from build123d import *

# Parameters (mm, degrees)
SKETCH1_W                   = 304.8
SKETCH1_H                   = 63.5
BOSS_EXTRUDE1_DEPTH         = 9.525
F_1_4_20_TAPPED_HOLE1_D     = 5.1054
F_1_4_0_25_DIAMETER_HOLE1_D = 6.35
F_8_32_TAPPED_HOLE1_D       = 3.4544
F_8_32_TAPPED_HOLE1_DEPTH   = 14.986
F_8_32_TAPPED_HOLE1_TIP     = 1.037806461


with BuildPart() as part:
    # Sketch1 → Boss-Extrude1 (new body)
    with BuildSketch(Plane.XY):
        Rectangle(SKETCH1_W, SKETCH1_H)
    extrude(amount=BOSS_EXTRUDE1_DEPTH)

    # 1/4-20 Tapped Hole1 (through all)
    with Locations(Plane(origin=(-41.275, 23.114, 9.525), x_dir=(1, 0, 0), z_dir=(0, 0, 1))):
        with Locations((0, 0), (82.55, 0), (82.55, -38.1), (0, -38.1)):
            Hole(F_1_4_20_TAPPED_HOLE1_D / 2)

    # 1/4 (0.25) Diameter Hole1 (through all)
    with Locations(Plane(origin=(-117.475, 22.225, 9.525), x_dir=(1, 0, 0), z_dir=(0, 0, 1))):
        with Locations((0, 0), (0, -44.323), (234.823, -44.323), (234.823, 0)):
            Hole(F_1_4_0_25_DIAMETER_HOLE1_D / 2)

    # #8-32 Tapped Hole1
    with Locations(Plane(origin=(-139.7, 31.75, 4.445), x_dir=(0, 0, 1), z_dir=(0, 1, 0))):
        with Locations((0, 0), (0, 279.4)):
            Hole(F_8_32_TAPPED_HOLE1_D / 2, depth=F_8_32_TAPPED_HOLE1_DEPTH)
            with Locations((0, 0, -(F_8_32_TAPPED_HOLE1_DEPTH + F_8_32_TAPPED_HOLE1_TIP / 2))):  # 118° drill point
                Cone(0, F_8_32_TAPPED_HOLE1_D / 2, F_8_32_TAPPED_HOLE1_TIP, mode=Mode.SUBTRACT)


solid = part.part
Verification items for the finished model (mm, model axes). Round coordinates to 2 decimals unless told otherwise and drop trailing zeros. Order: outer loops, then holes, each group sorted by start corner. A loop starts at its lowest first (then second) coordinate and runs counter-clockwise, first axis right, second up. Notation, with made-up numbers: (-11.75, -4.5) -> (36.25, -4.5) arc R20 ccw to (36.25, 15.5) -> close; hole circle Ø3 at (36, 49.5). An arc over 180 degrees is marked (long way). Put each result on its own line as item: value.
1) Mould release check, pull along X, two halves, no side actions. Record for faces 1 (the flat face through (-2, -31.75, 5)), 2 (the flat face through (-152.4, 0, 5)), 3 (the cylindrical face through (38.84, -14.22, 4.7)): +X half, -X half, draft (parallel to the pull), parting line (faces both ways), or undercut.
Final values:
face 1: draft
face 2: -X half
face 3: undercut
2) Depth check by flat-ended pin: pin 1 (6 mm diameter, centred on x = 41.275, y = 23.114, fed in from +Z) (3 decimals); pin 2 (3 mm diameter, centred on x = -139.7, z = 4.445, fed in from +Y). Enter the tip coordinate at first touch or a pass-through.
Final values:
pin 1: stops at z = 9.525
pin 2: stops at y = 16.63
3) Section check A-A (x = 117.5). Record the cut outline in (y, z) (3 decimals).
Final values:
outline: (-31.75, 0) -> (-25.269, 0) -> (-25.269, 9.525) -> (-31.75, 9.525) -> close; (-18.927, 0) -> (19.054, 0) -> (19.054, 9.525) -> (-18.927, 9.525) -> close; (25.396, 0) -> (31.75, 0) -> (31.75, 9.525) -> (25.396, 9.525) -> close
4) Material ranges on line 1 (X direction, y = -15, z = 8.5); line 2 (X direction, y = 26, z = 4.75); line 3 (Z direction, x = -139.7, y = 21.75) (3 decimals), recorded low to high.
Final values:
line 1: x = -152.4 to -43.83, -38.72 to 38.72, 43.83 to 152.4
line 2: x = -152.4 to -141.4, -138 to 138, 141.4 to 152.4
line 3: z = 0 to 2.718, 6.172 to 9.525
